Verification items for the finished model (mm, model axes). Give positions to 0.01 mm unless a question says otherwise; leave off trailing zeros. Write each loop counter-clockwise with the first axis right and the second up, starting at its lowest first coordinate (ties: lowest second). Pieces come first, ordered by that corner, then holes. Notation, with made-up numbers: (70.5, -33) - (91.5, -33) arc R16 cw to (91.5, -10) - close; hole circle Ø4 at (44, 47). An arc over 180 degrees is marked (long way). Answer as a JSON object with one key per item and string values. Group by question number.
Item 1: Sectioned sample at A-A, the plane z = 6.5. Record the boundary of the cut face in (x, y), and give its area (3 significant figures).
Item 2: Sectioned sample at B-B, the plane x = 485.5. Record the boundary of the cut face in (y, z).
Item 3: Sectioned sample at C-C, the plane y = 363.5. Record the boundary of the cut face in (x, z), and give its area (3 significant figures).
Item 4: Scan lines: line 1 along Y through (x, z) = (13.5, 6.25); line 2 along Y through (x, z) = (579, 7.75); line 3 along X through (y, z) = (30, 2.5). Record each from-to range of solid material in increasing order. Write a range as [from, to].
Item 5: Go/stop test with flat-tipped pins: pin 1 (1 mm diameter, centred on x = -329, z = 5, fed in from -Y); pin 2 (3 mm diameter, centred on x = -433.5, z = 9, fed in from -Y); pin 3 (5 mm diameter, centred on y = 315, z = 8, fed in from +X). Record where each tip stops, or that it passes through.
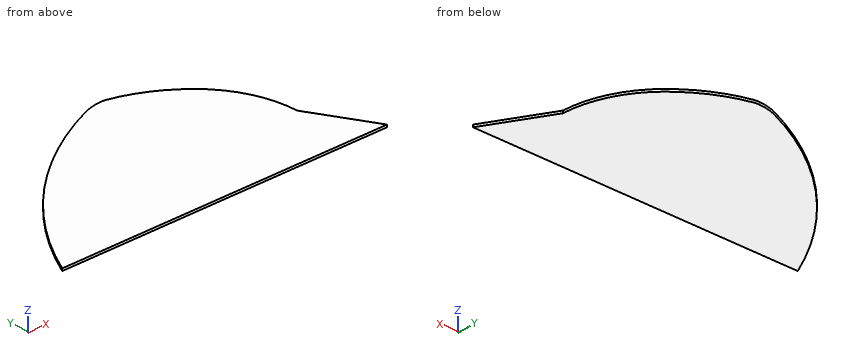
```python
from build123d import *

# Parameters (mm, degrees)
Y_KSEKLIK_EKSTR_ZYON1_DEPTH = 10


with BuildPart() as part:
    # Çizim1 → Yükseklik-Ekstrüzyon1 (new body)
    with BuildSketch(Plane.XY):
        with BuildLine():
            ThreePointArc((15.900247885, 707.260051266), (-426.128478979, 427.588769164), (-735.852954334, 6.072256116))
            Line((-735.852954334, 6.072256116), (664.147045666, -10.43069172))
            Line((664.147045666, -10.43069172), (514.004259651, 251.779036937))
            ThreePointArc((514.004259651, 251.779036937), (464.852209342, 449.785422775), (333.892309545, 606.22057716))
            ThreePointArc((333.892309545, 606.22057716), (228.125604356, 674.012353772), (110.348718239, 717.726493351))
            ThreePointArc((110.348718239, 717.726493351), (99.634050041, 719.676084087), (88.753877168, 720.152379041))
            ThreePointArc((88.753877168, 720.152379041), (51.840168654, 716.457617872), (15.900247885, 707.260051266))
        make_face()
    extrude(amount=Y_KSEKLIK_EKSTR_ZYON1_DEPTH)


solid = part.part
```
Geometry check:
{
 "1": {"outline": "(-735.85, 6.07) - (664.15, -10.43) - (514, 251.78) arc R453.58 ccw to (333.89, 606.22) arc R586.55 ccw to (110.35, 717.73) arc R80 ccw to (88.75, 720.15) arc R246.28 ccw to (15.9, 707.26) arc R1410.55 ccw to start", "area": "664,000 mm^2"},
 "2": {"outline": "(-8.32, 0) - (402.73, 0) - (402.73, 10) - (-8.32, 10) - close"},
 "3": {"outline": "(-490.55, 0) - (498.12, 0) - (498.12, 10) - (-490.55, 10) - close", "area": "9,890 mm^2"},
 "4": {"line 1": "[-2.76, 706.31]", "line 2": "[-9.43, 138.27]", "line 3": "[-724.1, 641]"},
 "5": {"pin 1": "y = 1.27", "pin 2": "y = 2.49", "pin 3": "x = 508.91"}
}
